Could you check a few things on this model? Use its own coordinates, in mm. Face numbers are marked on the shaded views. A direction names the side the tool comes from. Round coordinates to 2 decimals unless told otherwise and drop trailing zeros. Order: outer loops, then holes, each group sorted by start corner. A loop starts at its lowest first (then second) coordinate and runs counter-clockwise, first axis right, second up. Notation, with made-up numbers: (32, 76) - (37, 76) arc R15 cw to (37, 99) - close; hole circle Ø10 at (26.25, 21.5). An arc over 180 degrees is marked (long way). Return JSON: item names as keys, results as strings. Group by question number.
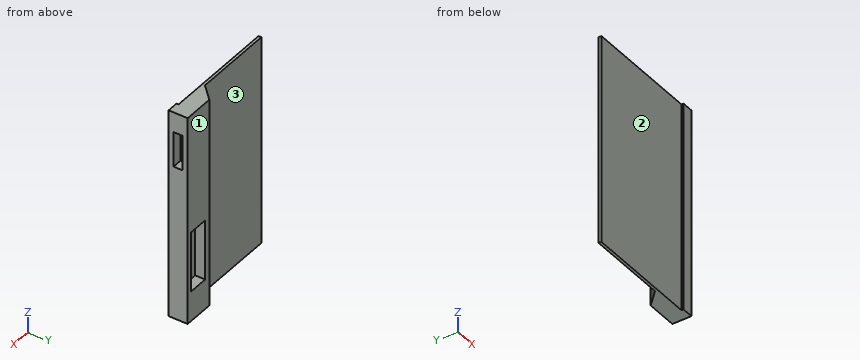
Autodesk Inventor part; units mm, degrees
ref_plane "YZ Plane" through (0, 0, 0) normal (1, 0, 0) x (0, 1, 0)
ref_plane "XZ Plane" through (0, 0, 0) normal (0, 1, 0) x (-1, 0, 0)
ref_plane "XY Plane" through (0, 0, 0) normal (0, 0, 1) x (1, 0, 0)
sketch "Sketch1" plane through (0, 0, 0) normal (0, 1, 0) x (-1, 0, 0)
  line L0 (-40.1461, 220.4385) -> (-360.1461, 220.4385)
  line L1 (-360.1461, 220.4385) -> (-360.1461, -309.5615)
  line L2 (-360.1461, -309.5615) -> (-40.1461, -309.5615)
  line L3 (-40.1461, -309.5615) -> (-40.1461, 220.4385)
  point P0 (0, 0)
  dimension "d0" = 530
  dimension "d1" = 320
extrude "Extrusion1" add sketch "Sketch1" along normal blind 7
sketch "Sketch7" plane through (0, 0, 0) normal (0, -1, 0) x (1, 0, 0)
  line L0 (360.1461, 220.4385) -> (360.1461, -309.5615)
  line L1 (40.1461, 220.4385) -> (360.1461, 220.4385)
  line L2 (360.1461, -309.5615) -> (331.5711, -309.5615)
  line L3 (331.5711, -309.5615) -> (331.5711, 220.4385)
  line L4 (331.5711, 220.4385) -> (360.1461, 220.4385)
  line L5 (360.1461, 220.4385) -> (360.1461, -309.5615)
  point P0 (0, 0)
  dimension "d15" = 28.575
extrude "Extrusion5" add sketch "Sketch7" along normal blind 5.08
sketch "Sketch8" plane through (0, 7, 0) normal (0, 1, 0) x (1, 0, 0)
  line L0 (360.1461, -220.4385) -> (360.1461, 309.5615)
  line L1 (360.1461, 309.5615) -> (40.1461, 309.5615)
  line L2 (360.1461, -220.4385) -> (283.9461, -220.4385)
  line L3 (283.9461, -220.4385) -> (283.9461, 309.5615)
  line L4 (283.9461, 309.5615) -> (360.1461, 309.5615)
  line L5 (360.1461, 309.5615) -> (360.1461, -220.4385)
  point P0 (0, 0)
  dimension "d18" = 76.2
extrude "Extrusion6" add sketch "Sketch8" along normal blind 36.068
sketch "Sketch9" plane through (0, 7, 0) normal (0, 1, 0) x (1, 0, 0)
  line L0 (283.9461, 309.5615) -> (283.9461, -220.4385)
  line L1 (283.9461, 309.5615) -> (40.1461, 309.5615)
  line L2 (283.9461, -220.4385) -> (245.8461, -220.4385)
  line L3 (245.8461, -220.4385) -> (245.8461, 309.5615)
  line L4 (245.8461, 309.5615) -> (283.9461, 309.5615)
  line L5 (283.9461, 309.5615) -> (283.9461, -220.4385)
  point P0 (0, 0)
  dimension "d21" = 38.1
extrude "Extrusion7" add sketch "Sketch9" along normal blind 36.068
chamfer "Chamfer1" distance 35.56 angle 45 1 edges at (245.8461, 43.068, -44.5615) measured on face at (245.8461, 19.0227, -132.8949)
sketch "Sketch10" plane through (0, 43.068, 0) normal (0, 1, 0) x (1, 0, 0)
  line L0 (296.6461, 80.9615) -> (347.4461, 80.9615)
  line L1 (347.4461, 80.9615) -> (347.4461, 233.3615)
  line L2 (347.4461, 233.3615) -> (296.6461, 233.3615)
  line L3 (296.6461, 233.3615) -> (296.6461, 80.9615)
  line L4 (360.1461, 309.5615) -> (281.4061, 309.5615)
  line L5 (360.1461, -220.4385) -> (360.1461, 309.5615)
  point P0 (0, 0)
  dimension "d27" = 76.2
  dimension "d28" = 228.6
  dimension "d29" = 12.7
  dimension "d30" = 63.5
extrude "Extrusion8" cut sketch "Sketch10" against normal blind 25.4
sketch "Sketch11" plane through (360.1461, -5.08, 220.4385) normal (1, 0, 0) x (0, 0, -1)
  line L0 (530, 12.588) -> (0, 12.588)
  line L1 (50.8, 35.56) -> (139.7, 35.56)
  line L2 (139.7, 35.56) -> (139.7, 12.588)
  line L3 (139.7, 12.588) -> (50.8, 12.588)
  line L4 (50.8, 12.588) -> (50.8, 35.56)
  line L5 (0, 48.148) -> (0, 0)
  line L6 (530, 0) -> (0, 0)
  line L7 (0, 48.148) -> (530, 48.148)
  point P0 (220.4385, 5.08)
  dimension "d33" = 50.8
  dimension "d34" = 139.7
  dimension "d35" = 12.588
  dimension "d36" = 12.588
extrude "Extrusion9" cut sketch "Sketch11" against normal blind 25.4
ref_plane "Work Plane2" through (185.8586, 0, -309.5615) normal (-1, 0, 0) x (0, 0, 1)
equation "\"d36\" = d35"
properties part number "Mock Acer SB230"
1) I want a section at B-B, the plane x = 192. List the corners of the cut face in (y, z) for me.
2) For the marked faces 1, 2 and 3, which set-ups out of +Z, -Z, +X, -X, +Y, -Y let a thin tool reach every point of the face, with its end or its side?
3) Will these pins go through, and if not, where does the flat tip stop? pin 1 (11.5 mm diameter, centred on y = 18.5, z = 135, fed in from +X); pin 2 (2 mm diameter, centred on x = 241, z = -132, fed in from +Y); pin 3 (1 mm diameter, centred on y = 11.5, z = -243.5, fed in from -X).
4) I want a section at A-A, the plane z = -197. List the corners of the cut face in (x, y) for me, plus the area to 3 significant figures.
5) If I drill on line 1 along Y through (x, z) = (338, 96); line 2 along Z through (x, y) = (317.5, 41); line 3 along Y through (x, z) = (187, -266.5), over which ranges is the centre line in solid material (lowest first)? Write a range as from..to.
6) I want a section at C-C, the plane x = 287. List the corners of the cut face in (y, z) for me.
Outcome:
{
 "1": {"outline": "(0, -309.56) - (7, -309.56) - (7, 220.44) - (0, 220.44) - close"},
 "2": {"face 1": "+Z, -Z, +X, -X, +Y", "face 2": "+Z, -Z, -X, -Y", "face 3": "+Z, -Z, -X, +Y"},
 "3": {"pin 1": "x = 334.75", "pin 2": "y = 7", "pin 3": "x = 249.34"},
 "4": {"outline": "(40.15, 0) - (331.57, 0) - (331.57, -5.08) - (360.15, -5.08) - (360.15, 43.07) - (347.45, 43.07) - (347.45, 17.67) - (296.65, 17.67) - (296.65, 43.07) - (281.41, 43.07) - (245.85, 7.51) - (245.85, 7) - (40.15, 7) - close", "area": "4,590 mm^2"},
 "5": {"line 1": "-5.08..7.51, 30.48..43.07", "line 2": "-309.56..-233.36, -80.96..220.44", "line 3": "0..7"},
 "6": {"outline": "(0, -309.56) - (43.07, -309.56) - (43.07, 220.44) - (0, 220.44) - close"}
}
